Here's the drawing with two shaded views (mm, measured from the low corner). I have some questions. Coordinates: 2 decimals unless noted, no trailing zeros. Write each loop counter-clockwise with the first axis right and the second up, starting at its lowest first coordinate (ties: lowest second). Pieces come first, ordered by that corner, then holes.
Item 1: I'm going to push a flat-ended pin straight in: pin 1 Ø5 at (x, z) = (7.5, 13) entering from -Y. Where does the tip first touch, or does it pass through?
Item 2: If we section it at A-A (z = 15): Please give me the cut outline in (x, y).
Item 3: If I drill on line 1 (Y direction, x = 5.5, z = 15); line 2 (Z direction, x = 4.5, y = 21); line 3 (Z direction, x = 2.25, y = 22), over which ranges is the centre line in solid material (lowest first)?
Item 4: We'd pull the mould along Y, two halves only. Please class the marked faces 1, 2 and 3: +Y half, -Y half, draft (parallel to the pull), parting line (faces both ways), or undercut.
Item 5: If we section it at B-B (y = 25): Please give me the cut outline in (x, z).
Item 6: If we section it at C-C (x = 1): Please give me the cut outline in (y, z).
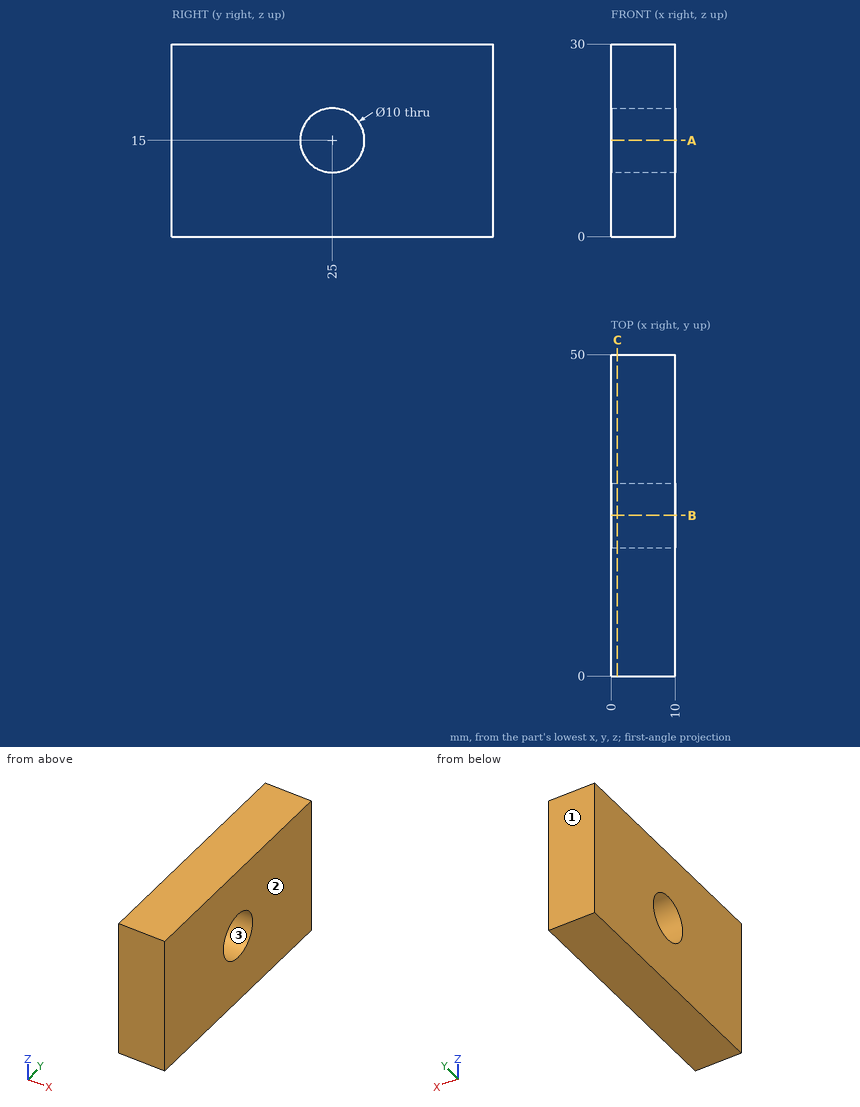
Answer list:
1. pin 1: stops at y = 0
2. outline: (0, 0) - (10, 0) - (10, 20) - (0, 20) - close; (0, 30) - (10, 30) - (10, 50) - (0, 50) - close
3. line 1: y = 0 to 20, 30 to 50
3. line 2: z = 0 to 12, 18 to 30
3. line 3: z = 0 to 11, 19 to 30
4. face 1: +Y half
4. face 2: draft
4. face 3: undercut
5. outline: (0, 0) - (10, 0) - (10, 10) - (0, 10) - close; (0, 20) - (10, 20) - (10, 30) - (0, 30) - close
6. outline: (0, 0) - (50, 0) - (50, 30) - (0, 30) - close; hole circle Ø10 at (25, 15)
